from build123d import *

# Parameters (mm, degrees)
F1_DEPTH      = 355.6
F3_DEPTH      = 19.051
F4_R          = 7.9375
F4_R_2        = 6.35
F5_DEPTH      = 3.175
F5_DEPTH_BACK = 22.225
F6_R          = 3.175
F7_DEPTH      = 1.0668


with BuildPart() as f1:
    # F0 (on Top) → F1 (new body)
    with BuildSketch(Plane.XY):
        with BuildLine():
            Line((-6.35, -9.525), (6.35, -9.525))
            ThreePointArc((6.35, -9.525), (8.595064, -8.595064), (9.525, -6.35))
            Line((9.525, -6.35), (9.525, 6.35))
            ThreePointArc((9.525, 6.35), (8.595064, 8.595064), (6.35, 9.525))
            Line((6.35, 9.525), (-6.35, 9.525))
            ThreePointArc((-6.35, 9.525), (-8.595064, 8.595064), (-9.525, 6.35))
            Line((-9.525, 6.35), (-9.525, -6.35))
            ThreePointArc((-9.525, -6.35), (-8.595064, -8.595064), (-6.35, -9.525))
        make_face()
        with BuildLine():
            ThreePointArc((-5.9182, -8.4582), (-7.714251, -7.714251), (-8.4582, -5.9182))
            Line((-8.4582, -5.9182), (-8.4582, 5.9182))
            ThreePointArc((-8.4582, 5.9182), (-7.714251, 7.714251), (-5.9182, 8.4582))
            Line((-5.9182, 8.4582), (5.9182, 8.4582))
            ThreePointArc((5.9182, 8.4582), (7.714251, 7.714251), (8.4582, 5.9182))
            Line((8.4582, 5.9182), (8.4582, -5.9182))
            ThreePointArc((8.4582, -5.9182), (7.714251, -7.714251), (5.9182, -8.4582))
            Line((5.9182, -8.4582), (-5.9182, -8.4582))
        make_face(mode=Mode.SUBTRACT)
    extrude(amount=F1_DEPTH)

    # F2 (on face) → F3 (cut, through all)
    with BuildSketch(Plane.YZ.offset(9.525)):
        with BuildLine():
            Line((-6.35, 122.2375), (-6.35, 131.7625))
            ThreePointArc((-6.35, 131.7625), (-7.9375, 127), (-6.35, 122.2375))
        make_face()
        with BuildLine():
            ThreePointArc((6.35, 122.2375), (7.530174, 124.489942), (7.9375, 127))
            ThreePointArc((7.9375, 127), (7.530174, 129.510058), (6.35, 131.7625))
            Line((6.35, 131.7625), (6.35, 122.2375))
        make_face()
        with BuildLine():
            Line((6.35, 122.2375), (6.35, 131.7625))
            ThreePointArc((6.35, 131.7625), (0, 134.9375), (-6.35, 131.7625))
            Line((-6.35, 131.7625), (-6.35, 122.2375))
            ThreePointArc((-6.35, 122.2375), (0, 119.0625), (6.35, 122.2375))
        make_face()
    extrude(amount=-F3_DEPTH, mode=Mode.SUBTRACT)

    # F4 (on face) → F5 (join, two sides)
    with BuildSketch(Plane.YZ.offset(9.525)) as f5_sk:
        with Locations((0, 127)):
            Circle(F4_R)
        with Locations((0, 127)):
            Circle(F4_R_2, mode=Mode.SUBTRACT)
    extrude(amount=F5_DEPTH)
    extrude(f5_sk.sketch, amount=-F5_DEPTH_BACK)

    # F6 (on face) → F7 (join)
    with BuildSketch(Plane.YZ.offset(9.525)):
        with BuildLine():
            Line((-25.4, 0), (6.35, 0))
            Line((6.35, 0), (6.35, 110.897045))
            Line((6.35, 110.897045), (-28.575, 90.733087))
            ThreePointArc((-28.575, 90.733087), (-30.899261, 88.408826), (-31.75, 85.233826))
            Line((-31.75, 85.233826), (-31.75, 6.35))
            ThreePointArc((-31.75, 6.35), (-29.890128, 1.859872), (-25.4, 0))
        make_face()
        with Locations((-22.225, 7.874)):
            Circle(F6_R, mode=Mode.SUBTRACT)
        with Locations((-22.225, 18.542)):
            Circle(F6_R, mode=Mode.SUBTRACT)
        with Locations((-22.225, 29.21)):
            Circle(F6_R, mode=Mode.SUBTRACT)
        with Locations((-22.225, 39.878)):
            Circle(F6_R, mode=Mode.SUBTRACT)
        with Locations((-22.225, 50.546)):
            Circle(F6_R, mode=Mode.SUBTRACT)
        with Locations((-22.225, 61.214)):
            Circle(F6_R, mode=Mode.SUBTRACT)
        with Locations((-22.225, 71.882)):
            Circle(F6_R, mode=Mode.SUBTRACT)
        with Locations((-22.225, 82.55)):
            Circle(F6_R, mode=Mode.SUBTRACT)
    extrude(amount=F7_DEPTH)


solid = f1.part
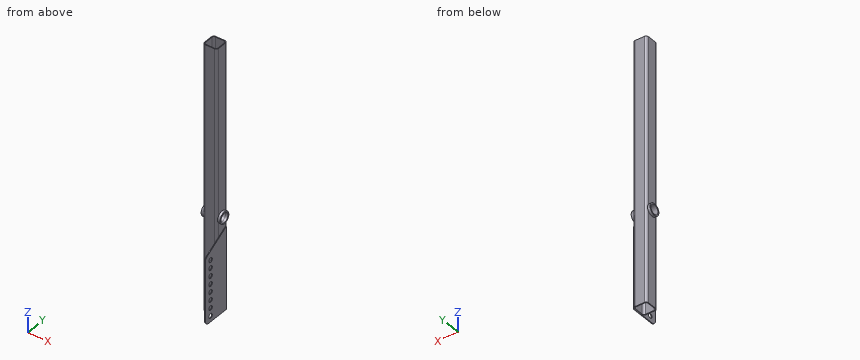
Read the model definition and answer for the solid it produces. Units are mm, in the model's axes. Round coordinates to 2 decimals unless told otherwise and drop trailing zeros. Loops run counter-clockwise (first coordinate to the right, second up) from the corner with the lowest first, then second, coordinate; pieces in that order, holes last. Notation, with made-up numbers: (78.25, 19) - (107.25, 19) arc R31 cw to (107.25, 43) - close; hole circle Ø4 at (57, 75). An arc over 180 degrees is marked (long way). One line per question, with ' | ' between items. Start each with the question number.
Q1. Section B-B on x = 3 is taken. Count the separate pieces of the cut face and the enclosed holes in it, plus the area to 3 significant figures.
Q2. Section A-A on z = 29.21 is taken. Give the vertices of the cut face in (x, y) (3 decimals), plus the area to 3 significant figures.
Q3. Flat-ended cylindrical pins translate along their axes: pin 1 (7.5 mm diameter, centred on y = -22.225, z = 18.542, fed in from +X); pin 2 (6 mm diameter, centred on x = -7.5, z = 273.5, fed in from +Y) (3 decimals); pin 3 (14 mm diameter, centred on y = 1.5, z = 59, fed in from -X) (3 decimals); pin 4 (7.5 mm diameter, centred on y = -25.5, z = 63.5, fed in from -X) (3 decimals). Find the tip coordinate at first contact, or state that the pin passes through.
Q4. Section C-C on z = 255.5 is taken. Give the vertices of the cut face in (x, y) (3 decimals), plus the area to 3 significant figures.
Q5. Find the intervals of material crossed by L1, parallel to Y at x = 5.25, z = 325.5 (3 decimals); L2, parallel to X at y = -4, z = 41 (3 decimals), in increasing order.
Established:
1) separate pieces: 3 | enclosed holes: 1 | area: 830 mm²
2) outline: (-9.525, -6.35) arc R3.175 ccw to (-6.35, -9.525) - (6.35, -9.525) arc R3.175 ccw to (9.525, -6.35) - (9.525, -19.05) - (10.592, -19.05) - (10.592, 6.35) - (9.525, 6.35) arc R3.175 ccw to (6.35, 9.525) - (-6.35, 9.525) arc R3.175 ccw to (-9.525, 6.35) - close; (9.525, -31.75) - (10.592, -31.75) - (10.592, -25.4) - (9.525, -25.4) - close; hole (-8.458, -5.918) arc R2.54 ccw to (-5.918, -8.458) - (5.918, -8.458) arc R2.54 ccw to (8.458, -5.918) - (8.458, 5.918) arc R2.54 ccw to (5.918, 8.458) - (-5.918, 8.458) arc R2.54 ccw to (-8.458, 5.918) - close | area: 107 mm²
3) pin 1: x = 10.59 | pin 2: y = 9.525 | pin 3: x = -9.525 | pin 4: x = 9.525
4) outline: (-9.525, -6.35) arc R3.175 ccw to (-6.35, -9.525) - (6.35, -9.525) arc R3.175 ccw to (9.525, -6.35) - (9.525, 6.35) arc R3.175 ccw to (6.35, 9.525) - (-6.35, 9.525) arc R3.175 ccw to (-9.525, 6.35) - close; hole (-8.458, -5.918) arc R2.54 ccw to (-5.918, -8.458) - (5.918, -8.458) arc R2.54 ccw to (8.458, -5.918) - (8.458, 5.918) arc R2.54 ccw to (5.918, 8.458) - (-5.918, 8.458) arc R2.54 ccw to (-8.458, 5.918) - close | area: 73.6 mm²
5) L1: -9.525 to -8.458, 8.458 to 9.525 | L2: -9.525 to -8.458, 8.458 to 10.592
